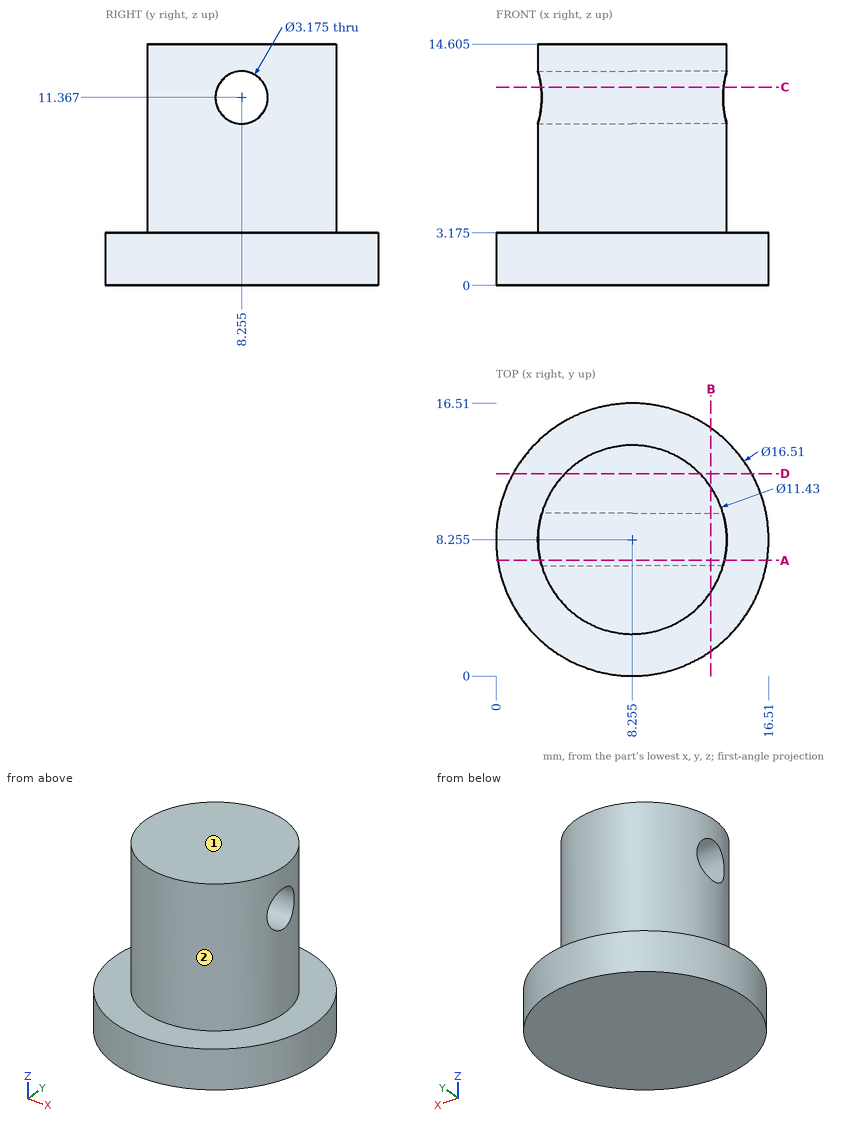
Answer from the drawing. Dimensions are ordinates in mm from the lowest x, y and z of the part. A direction names the side the tool comes from. Round coordinates to 2 decimals unless told otherwise and drop trailing zeros. Order: outer loops, then holes, each group sorted by start corner. A loop starts at its lowest first (then second) coordinate and runs counter-clockwise, first axis right, second up. Notation, with made-up numbers: (47, -38.75) - (88, -38.75) arc R7 cw to (88, -30.75) - close; hole circle Ø6 at (54.5, -36.5). An arc over 180 degrees is marked (long way). Put each result on its own line as item: value. Start each with the question number.
(1) Find section A-A (y = 7). Give the vertices of the cut face in (x, z) (1 decimal).
(2) Straight lines are drawn through the part: probe 1 along Z at (x, y) = (15, 12.75) (1 decimal); probe 2 along Z at (x, y) = (7.5, 8.5) (1 decimal); probe 3 along X at (y, z) = (8.25, 5). For each, find the intervals that lie inside material, in ascending order. Write a range as from..to.
(3) Given P1, Ø1, axis at y = 9.5, z = 9.5, coming from the +X side; P2, Ø4, axis at x = 14.5, z = 4.5, coming from the +Y side; P3, Ø4, axis at y = 8.26, z = 11.37, coming from the -X side; P4, Ø2.5, axis at y = 8.26, z = 11.37, coming from the +X side, each flat-ended and moving along its own axis, determine where each tip first touches the part or whether it passes through.
(4) Find section B-B (x = 13). Give the vertices of the cut face in (y, z) (1 decimal), plus the area to 3 significant figures.
(5) For the marked faces 1 and 2, determine the directions among +Z, -Z, +X, -X, +Y, -Y from which every point of the face is accessible in a straight line to the end or side of a thin tool.
(6) Find section D-D (y = 12.25). Give the vertices of the cut face in (x, z) (1 decimal).
(7) Find section C-C (z = 12). Give the vertices of the cut face in (x, y) (1 decimal).
Reply:
1. outline: (0.1, 0) - (16.4, 0) - (16.4, 3.2) - (13.8, 3.2) - (13.8, 10.4) - (2.7, 10.4) - (2.7, 3.2) - (0.1, 3.2) - close; (2.7, 12.3) - (13.8, 12.3) - (13.8, 14.6) - (2.7, 14.6) - close
2. probe 1: 0..3.2
2. probe 2: 0..9.8, 12.9..14.6
2. probe 3: 2.54..13.97
3. P1: x = 13.92
3. P2: y = 15.01
3. P3: x = 2.54
3. P4: through
4. outline: (1.5, 0) - (15, 0) - (15, 3.2) - (11.4, 3.2) - (11.4, 14.6) - (5.1, 14.6) - (5.1, 3.2) - (1.5, 3.2) - close; hole circle Ø3.2 at (8.3, 11.4)
4. area: 108 mm^2
5. face 1: +Z, +X, -X, +Y, -Y
5. face 2: +Z
6. outline: (1, 0) - (15.5, 0) - (15.5, 3.2) - (12.3, 3.2) - (12.3, 14.6) - (4.2, 14.6) - (4.2, 3.2) - (1, 3.2) - close
7. outline: (2.7, 6.8) arc R5.7 ccw to (13.8, 6.8) - close; (2.7, 9.7) - (13.8, 9.7) arc R5.7 ccw to start
